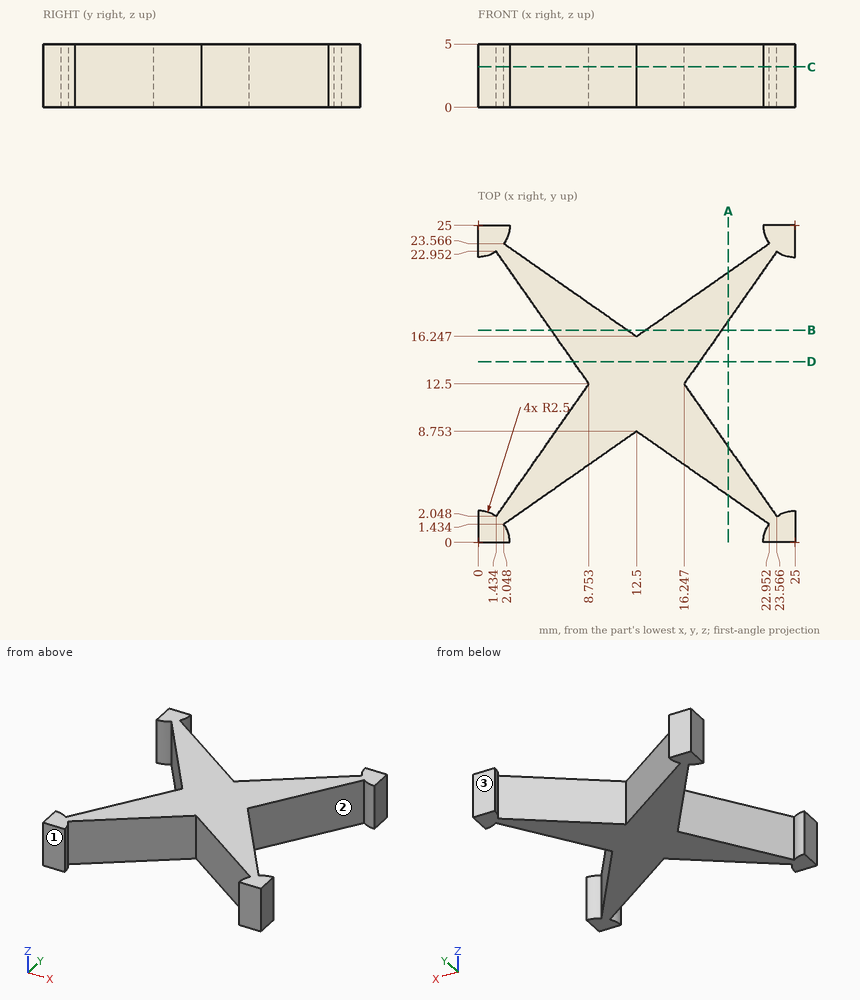
Drawing for the job (mm, zero at the part's lowest x, y, z). Give positions to 0.01 mm unless a question says otherwise; leave off trailing zeros. Loops run counter-clockwise (first coordinate to the right, second up) from the corner with the lowest first, then second, coordinate; pieces in that order, holes last. Notation, with made-up numbers: M 74,32.5 L 78,32.5 A22 cw 78,64.5 Z; hole C -2.75,43 d3. An arc over 180 degrees is marked long. One line per question, with ' | ' between items. Start each with the question number.
1. Two-plate mould, pull along Y, no slides. Class the marked faces 1, 2 and 3: pulls with the +Y half, pulls with the -Y half, needs draft (parallel to the pull), parting line crosses it, or undercut.
2. Flat gauge pins, fed straight in: pin 1 (1.5 mm diameter, centred on y = 7.5, z = 2, fed in from +X); pin 2 (3 mm diameter, centred on y = 20, z = 2, fed in from -X). Where does each tip first touch, or does it go through?
3. Saw through at D-D on y = 14.25. Give the cut face in (x, z).
4. Saw through at C-C on z = 3.2. Give the cut face in (x, y), plus the area to 3 significant figures.
5. Saw through at A-A on x = 19.75. Give the cut face in (y, z), plus the area to 3 significant figures.
6. Saw through at B-B on y = 16.75. Give the cut face in (x, z).
7. Probe L1, parallel to X at y = 8.5, z = 3.5; L2, parallel to Y at x = 3, z = 2.1 (1 decimal); L3, parallel to Y at x = 17.25, z = 3.7 (1 decimal). List the from-to ranges inside material, lowest first. Write a range as from..to.
Result sheet:
1) face 1: pulls with the -Y half | face 2: undercut | face 3: pulls with the +Y half
2) pin 1: stops at x = 20.27 | pin 2: stops at x = 2.45
3) outline: M 7.53,0 L 17.47,0 L 17.47,5 L 7.53,5 Z
4) outline: M 0,0 L 2.5,0 A2.5 ccw 2.05,1.43 L 12.5,8.75 L 22.95,1.43 A2.5 ccw 22.5,0 L 25,0 L 25,2.5 A2.5 ccw 23.57,2.05 L 16.25,12.5 L 23.57,22.95 A2.5 ccw 25,22.5 L 25,25 L 22.5,25 A2.5 ccw 22.95,23.57 L 12.5,16.25 L 2.05,23.57 A2.5 ccw 2.5,25 L 0,25 L 0,22.5 A2.5 ccw 1.43,22.95 L 8.75,12.5 L 1.43,2.05 A2.5 ccw 0,2.5 Z | area: 203 mm^2
5) outline: M 3.68,0 L 7.5,0 L 7.5,5 L 3.68,5 Z; M 17.5,0 L 21.32,0 L 21.32,5 L 17.5,5 Z | area: 38.2 mm^2
6) outline: M 5.78,0 L 11.78,0 L 11.78,5 L 5.78,5 Z; M 13.22,0 L 19.22,0 L 19.22,5 L 13.22,5 Z
7) L1: x = 5.95..12.14, 12.86..19.05 | L2: y = 2.1..4.3, 20.7..22.9 | L3: y = 5.4..11.1, 13.9..19.6
